```python
from build123d import *

# Parameters (mm, degrees)
ESQUISSE1_W             = 15
ESQUISSE1_H             = 15
ESQUISSE1_R             = 4.15
BOSS_EXTRU_1_DEPTH      = 15
ESQUISSE2_R             = 2.15
ENL_V_MAT_EXTRU_1_DEPTH = 8.5


with BuildPart() as part:
    # Esquisse1 → Boss.-Extru.1 (new body)
    with BuildSketch(Plane(origin=(0, 0, 0), x_dir=(1, 0, 0), z_dir=(0, 1, 0))):
        Rectangle(ESQUISSE1_W, ESQUISSE1_H)
        Circle(ESQUISSE1_R, mode=Mode.SUBTRACT)
    extrude(amount=BOSS_EXTRU_1_DEPTH)

    # Esquisse2 → Enlèv. mat.-Extru.1 (cut, through all)
    with BuildSketch(Plane.XY):
        with Locations((0, 7.5)):
            Circle(ESQUISSE2_R)
    extrude(amount=-ENL_V_MAT_EXTRU_1_DEPTH, mode=Mode.SUBTRACT)


solid = part.part
```
Geometry: final body of the model. Coordinates: model frame, mm. A direction names the side the tool comes from. Round coordinates to 2 decimals unless told otherwise and drop trailing zeros. Order: outer loops, then holes, each group sorted by start corner. A loop starts at its lowest first (then second) coordinate and runs counter-clockwise, first axis right, second up. Notation, with made-up numbers: (74.25, 40.25) -> (133.25, 40.25) arc R19 cw to (133.25, 74.25) -> close; hole circle Ø8 at (57, 32.5). An arc over 180 degrees is marked (long way). Use one line per item in the form item = value. Start each with the question number.
1. Cut plane D-D (z = -5). Return the cut outline in (x, y).
2. Draft query along X for faces 3 (the face through (-0.9, 7.4, 4.05)), 4 (the face through (-2, 9, -7.5)), 5 (the face through (-7.5, 7, 0)). Return one class per face: pulls with the +X half, pulls with the -X half, needs draft (parallel to the pull), parting line crosses it, or undercut.
3. Cut plane B-B (z = 0). Return the cut outline in (x, y), then the cut area to 4 significant figures.
4. Cut plane A-A (x = 0). Return the cut outline in (y, z), then the cut area to 3 significant figures.
5. Reachability of faces 1 (the face through (2.05, 8.15, -5.5)), 2 (the face through (-3.4, 15, -3.4)) from +Z, -Z, +X, -X, +Y, -Y: full face, straight path, thin tool, end or side. Return the list, or none.
6. Cut plane C-C (y = 7.5). Return the cut outline in (x, z), then the cut area to 3 significant figures.
7. Line query: probe 1 along X at (y, z) = (5, 0); probe 2 along X at (y, z) = (7.5, -5.6); probe 3 along Y at (x, z) = (0, -5.8). Output: solid intervals per line, ascending.
Solution:
q1.outline = (-7.5, 0) -> (7.5, 0) -> (7.5, 15) -> (-7.5, 15) -> close; hole circle Ø4.3 at (0, 7.5)
q2.face_3 = undercut
q2.face_4 = needs draft
q2.face_5 = pulls with the -X half
q3.outline = (-7.5, 0) -> (-4.15, 0) -> (-4.15, 15) -> (-7.5, 15) -> close; (4.15, 0) -> (7.5, 0) -> (7.5, 15) -> (4.15, 15) -> close
q3.area = 100.5 mm^2
q4.outline = (0, -7.5) -> (5.35, -7.5) -> (5.35, -4.15) -> (0, -4.15) -> close; (0, 4.15) -> (15, 4.15) -> (15, 7.5) -> (0, 7.5) -> close; (9.65, -7.5) -> (15, -7.5) -> (15, -4.15) -> (9.65, -4.15) -> close
q4.area = 86.1 mm^2
q5.face_1 = -Z
q5.face_2 = +Z, -Z, +X, -X, +Y
q6.outline = (-7.5, -7.5) -> (-2.15, -7.5) -> (-2.15, -3.55) arc R4.15 cw (long way) to (2.15, -3.55) -> (2.15, -7.5) -> (7.5, -7.5) -> (7.5, 7.5) -> (-7.5, 7.5) -> close
q6.area = 156 mm^2
q7.probe_1 = -7.5 to -4.15, 4.15 to 7.5
q7.probe_2 = -7.5 to -2.15, 2.15 to 7.5
q7.probe_3 = 0 to 5.35, 9.65 to 15
